Design review of the part built by this model. Coordinates are the model's own, in mm. Coordinates: 2 decimals unless noted, no trailing zeros. Loops run counter-clockwise (first coordinate to the right, second up) from the corner with the lowest first, then second, coordinate; pieces in that order, holes last. Notation, with made-up numbers: M 34.5,24.25 L 63.5,24.25 A24 ccw 63.5,45.25 Z; hole C 39,60.25 d9. An arc over 180 degrees is marked long. Answer as a JSON object with one key per item and string values. Group by question number.
1. Insertion check: pin 1 (5 mm diameter, centred on x = 28, z = 11.5, fed in from +Y); pin 2 (0.9 mm diameter, centred on x = 66.5, z = 3, fed in from -Y); pin 3 (6.5 mm diameter, centred on y = -56, z = 29.5, fed in from +X). Each pin has a flat end and moves straight along its axis. Give the tip position at first contact, or say it passes through.
2. Consider section B-B (x = 11). State the section outline as (y, z) points, then the cut area to 3 significant figures.
3. To check wall thickness, follow probe 1 along Z at (x, y) = (-39, -56.5); probe 2 along X at (y, z) = (-32, 3.5); probe 3 along X at (y, z) = (-54.8, 40). State the ranges of each line that lie inside material, in increasing order.
4. Consider section D-D (x = -39). State the section outline as (y, z) points, then the cut area to 3 significant figures.
5. Consider section A-A (z = 12). State the section outline as (x, y) points.
6. Consider section C-C (y = -4). State the section outline as (x, z) points, then the cut area to 4 significant figures.
Autodesk Inventor part; units mm, degrees
ref_plane "YZ Plane" through (0, 0, 0) normal (1, 0, 0) x (0, 1, 0)
ref_plane "XZ Plane" through (0, 0, 0) normal (0, 1, 0) x (-1, 0, 0)
ref_plane "XY Plane" through (0, 0, 0) normal (0, 0, 1) x (1, 0, 0)
sketch "Skizze1" plane through (0, 0, 0) normal (0, 0, 1) x (1, 0, 0)
  line L0 (-77, 59.5) -> (77, 59.5)
  line L1 (77, 59.5) -> (77, -59.5)
  line L2 (77, -59.5) -> (-77, -59.5)
  line L3 (-77, -59.5) -> (-77, 59.5)
  line L4 (-77, 59.5) -> (77, -59.5) construction
  line L5 (77, 59.5) -> (-77, -59.5) construction
  point P0 (0, 0)
  dimension "d0" = 154
  dimension "d1" = 119
extrude "Extrusion1" add sketch "Skizze1" along normal blind 5
fillet "Rundung1" radius 17 4 edges at (77, 59.5, 2.5) (77, -59.5, 2.5) (-77, -59.5, 2.5) (-77, 59.5, 2.5)
chamfer "Fasen1" distance 1.5 angle 45 8 edges at (-72.0208, 54.5208, 0) (-77, 0, 0) (-72.0208, -54.5208, 0) (0, -59.5, 0) (72.0208, -54.5208, 0) (77, 0, 0) (72.0208, 54.5208, 0) (0, 59.5, 0)
sketch "Skizze2" plane through (0, 0, 5) normal (0, 0, 1) x (1, 0, 0)
  line L0 (-55, 47.5) -> (55, 47.5)
  line L1 (65, 37.5) -> (65, -37.5)
  line L2 (55, -47.5) -> (-55, -47.5)
  line L3 (-65, -37.5) -> (-65, 37.5)
  line L4 (-65, 47.5) -> (65, -47.5) construction
  line L5 (65, 47.5) -> (-65, -47.5) construction
  arc A0 (-55, 47.5) -> (-65, 37.5) centre (-55, 37.5) ccw
  arc A1 (65, 37.5) -> (55, 47.5) centre (55, 37.5) ccw
  arc A2 (-65, -37.5) -> (-55, -47.5) centre (-55, -37.5) ccw
  arc A3 (55, -47.5) -> (65, -37.5) centre (55, -37.5) ccw
  line L6 (77, -42.5) -> (77, 42.5)
  line L7 (-77, 42.5) -> (-77, -42.5)
  line L8 (-60, -59.5) -> (60, -59.5)
  line L9 (60, 59.5) -> (-60, 59.5)
  point P0 (0, 0)
  dimension "d10" = 10
  dimension "d11" = 10
  dimension "d12" = 10
  dimension "d13" = 10
  dimension "d14" = 95
  dimension "d15" = 130
  dimension "d16" = 154
  dimension "d17" = 119
extrude "Extrusion2" cut sketch "Skizze2" against normal through all
sketch "Skizze3" plane through (0, 0, 5) normal (0, 0, 1) x (1, 0, 0)
  line L0 (-71.5, 44) -> (71.5, 44)
  line L1 (71.5, 44) -> (71.5, -44)
  line L2 (71.5, -44) -> (-71.5, -44)
  line L3 (-71.5, -44) -> (-71.5, 44)
  line L4 (-71.5, 44) -> (71.5, -44) construction
  line L5 (71.5, 44) -> (-71.5, -44) construction
  point P0 (0, 0)
  dimension "d20" = 143
  dimension "d21" = 88
extrude "Extrusion3" cut sketch "Skizze3" against normal blind 3
sketch "Skizze5" plane through (0, 0, 5) normal (0, 0, 1) x (1, 0, 0)
  line L0 (-77, 42.5) -> (-77, -42.5)
  line L1 (-35, -59.5) -> (-43, -59.5)
  line L2 (-43, -59.5) -> (-43, -53.6)
  line L3 (-43, -53.6) -> (-35, -53.6)
  line L4 (-35, -53.6) -> (-35, -59.5)
  line L5 (-35, -59.5) -> (-43, -53.6) construction
  line L6 (-43, -59.5) -> (-35, -53.6) construction
  line L7 (-60, -59.5) -> (60, -59.5)
  line L8 (30, -59.5) -> (22, -59.5)
  line L9 (22, -59.5) -> (22, -53.6)
  line L10 (22, -53.6) -> (30, -53.6)
  line L11 (30, -53.6) -> (30, -59.5)
  line L12 (30, -59.5) -> (22, -53.6) construction
  line L13 (22, -59.5) -> (30, -53.6) construction
  point P0 (0, 0)
  point P1 (-39, -56.55)
  point P2 (26, -56.55)
  dimension "d29" = 38
  dimension "d30" = 5.9
  dimension "d31" = 8
  dimension "d37" = 103
  dimension "d38" = 8
  dimension "d39" = 5.9
extrude "Extrusion5" add sketch "Skizze5" along normal blind 40 contours L1 L2 L3 L4
chamfer "Fasen2" distance 10 angle 45 2 edges at (-43, -56.55, 5) (-35, -56.55, 5)
sketch "Skizze6" plane through (0, 0, 5) normal (0, 0, 1) x (1, 0, 0)
  line L0 (22, -53.6) -> (30, -53.6)
  line L1 (30, -53.6) -> (30, -59.5)
  line L2 (30, -59.5) -> (22, -59.5)
  line L3 (22, -59.5) -> (22, -53.6)
  point P0 (0, 0)
extrude "Extrusion6" add sketch "Skizze6" along normal blind 10.5
chamfer "Fasen3" distance 5 angle 45 2 edges at (22, -56.55, 5) (30, -56.55, 5)
sketch "Skizze7" plane through (0, 0, 2) normal (0, 0, 1) x (1, 0, 0)
  line L0 (-65, -27) -> (-70, -27)
  line L1 (-70, -27) -> (-70, -19)
  line L2 (-70, -19) -> (-65, -19)
  line L3 (-65, -19) -> (-65, -27)
  line L4 (-65, -27) -> (-70, -19) construction
  line L5 (-70, -27) -> (-65, -19) construction
  line L6 (-62.5993, -44) -> (-71.5, -44)
  line L7 (-65, 37.5) -> (-65, -37.5)
  point P0 (0, 0)
  point P1 (-67.5, -23)
  dimension "d45" = 21
  dimension "d46" = 8
  dimension "d48" = 5
extrude "Extrusion7" cut sketch "Skizze7" against normal blind 3
sketch "Skizze8" plane through (22, -53.6, 15.5) normal (0, 1, 0) x (1, 0, 0)
  line L0 (-57, -29.5) -> (-65, -29.5)
  circle A0 centre (-61, -24.5) radius 2
  circle A1 centre (-61, -6.5) radius 2
  circle A2 centre (4, 3.5) radius 2
  line L1 (8, 0) -> (0, 0)
  line L2 (-61, -29.5) -> (-61, 10.5) construction
  line L3 (-77, 10.5) -> (33, 10.5) construction
  point P0 (-22, 15.5)
  point P1 (4, 0)
  dimension "d51" = 4
  dimension "d52" = 5
  dimension "d53" = 4
  dimension "d54" = 18
  dimension "d55" = 4
  dimension "d56" = 33
  dimension "d57" = 0
extrude "Extrusion8" cut sketch "Skizze8" against normal through all
properties part number "220_Frame_Mainboard"
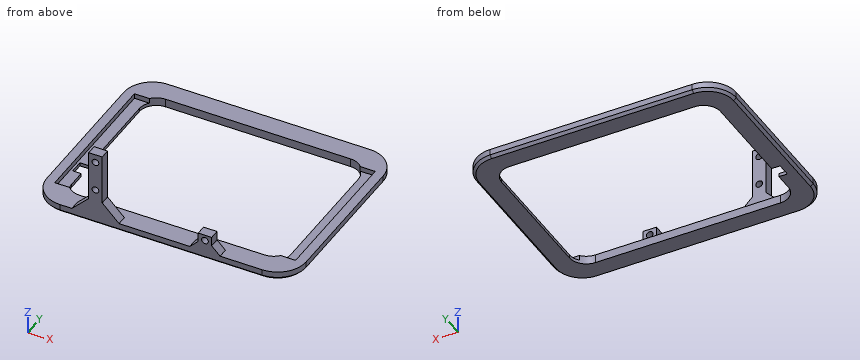
Findings below:
{
 "1": {"pin 1": "stops at y = -53.6", "pin 2": "stops at y = -58.39", "pin 3": "stops at x = -35"},
 "2": {"outline": "M -59.5,1.5 L -58,0 L -47.5,0 L -47.5,5 L -59.5,5 Z; M 47.5,0 L 58,0 L 59.5,1.5 L 59.5,5 L 47.5,5 Z", "area": "118 mm^2"},
 "3": {"probe 1": "z = 0 to 20, 24 to 38, 42 to 45", "probe 2": "x = -77 to -71.5, 71.5 to 77", "probe 3": "x = -43 to -41, -37 to -35"},
 "4": {"outline": "M -59.5,1.5 L -58,0 L -47.5,0 L -47.5,5 L -53.6,5 L -53.6,20 L -59.5,20 Z; M -59.5,24 L -53.6,24 L -53.6,38 L -59.5,38 Z; M -59.5,42 L -53.6,42 L -53.6,45 L -59.5,45 Z; M 47.5,0 L 58,0 L 59.5,1.5 L 59.5,5 L 47.5,5 Z", "area": "307 mm^2"},
 "5": {"outline": "M -46,-59.5 L -32,-59.5 L -32,-53.6 L -46,-53.6 Z; M 22,-59.5 L 24,-59.5 L 24,-53.6 L 22,-53.6 Z; M 28,-59.5 L 30,-59.5 L 30,-53.6 L 28,-53.6 Z"},
 "6": {"outline": "M -77,1.5 L -75.5,0 L -65,0 L -65,2 L -71.5,2 L -71.5,5 L -77,5 Z; M 65,0 L 75.5,0 L 77,1.5 L 77,5 L 71.5,5 L 71.5,2 L 65,2 Z", "area": "78.75 mm^2"}
}
